Verification items for this drawing (mm, ordinates from the low corner). A direction names the side the tool comes from. Round coordinates to 2 decimals unless told otherwise and drop trailing zeros. Order: outer loops, then holes, each group sorted by start corner. A loop starts at its lowest first (then second) coordinate and runs counter-clockwise, first axis right, second up. Notation, with made-up numbers: (-25, -22.75) -> (16, -22.75) arc R13 cw to (16, -15.75) -> close; hole circle Ø1 at (-6, 81.5). An arc over 180 degrees is marked (long way). Answer in a Markdown table with one row per item. Add a question column.
1. Sectioned sample at C-C, the plane y = 10.5. Record the boundary of the cut face in (x, z), then the cut area to 3 significant figures.
2. Draft check along X on the marked faces 1, 2 and 3. Enter one of: +X half, -X half, draft (parallel to the pull), parting line (faces both ways), or undercut.
3. Depth check by flat-ended pin: P1, Ø7.5, axis at x = 53, y = 36, coming from the +Z side; P2, Ø1, axis at x = 38.5, z = 111.5, coming from the -Y side; P3, Ø6.5, axis at x = 69, y = 35, coming from the +Z side. Enter the tip coordinate at first touch or a pass-through.
4. Sectioned sample at B-B, the plane z = 98.5. Record the boundary of the cut face in (x, y), then the cut area to 3 significant figures.
5. Access from +Z, -Z, +X, -X, +Y, -Y to the whole of each face (thin tool, end or side, straight path). Record for the marked faces 4 and 5.
6. Material ranges on L1, parallel to X at y = 8.5, z = 69; L2, parallel to Z at x = 51, y = 37; L3, parallel to X at y = 24, z = 111.5, recorded low to high. Write a range as from..to.
7. Sectioned sample at A-A, the plane z = 118. Record the boundary of the cut face in (x, y), then the cut area to 3 significant figures.
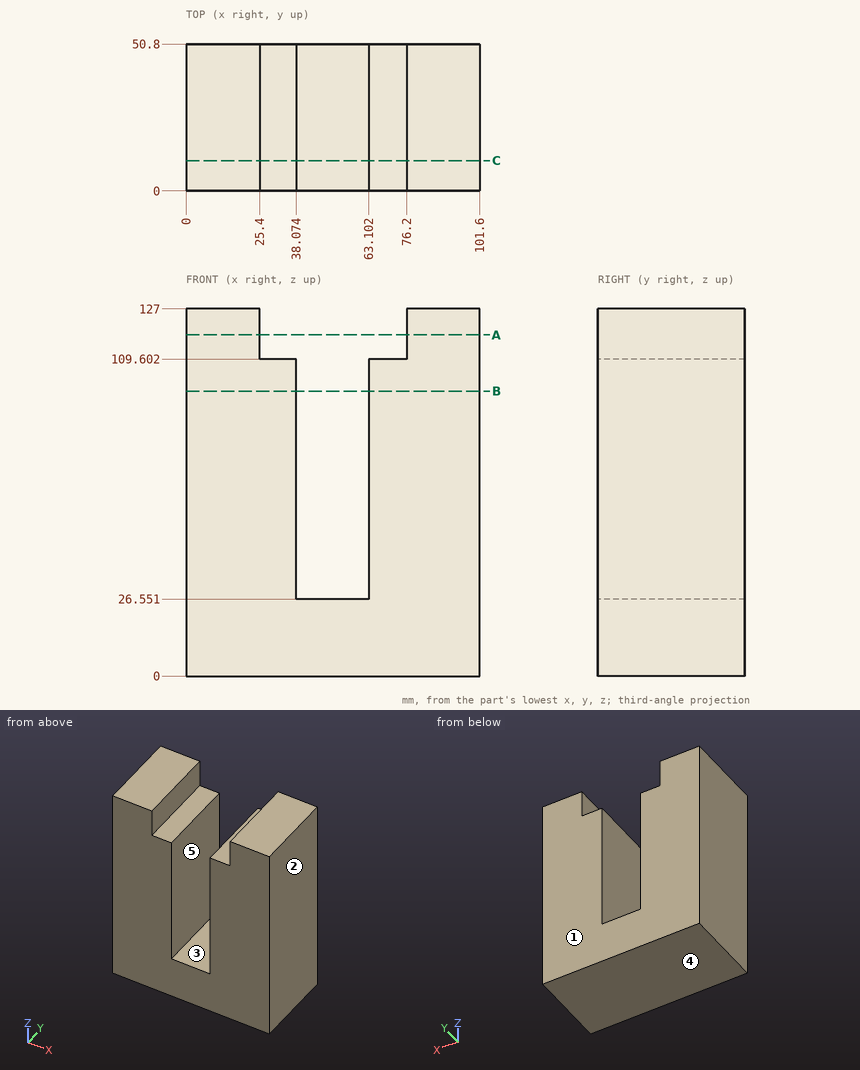
Answer key:
| question | item | result |
|---|---|---|
| 1 | outline | (0, 0) -> (101.6, 0) -> (101.6, 127) -> (76.2, 127) -> (76.2, 109.6) -> (63.1, 109.6) -> (63.1, 26.55) -> (38.07, 26.55) -> (38.07, 109.6) -> (25.4, 109.6) -> (25.4, 127) -> (0, 127) -> close |
| 1 | area | 9,940 mm² |
| 2 | face 1 | draft |
| 2 | face 2 | +X half |
| 2 | face 3 | undercut |
| 3 | P1 | stops at z = 26.55 |
| 3 | P2 | passes through |
| 3 | P3 | stops at z = 109.6 |
| 4 | outline | (0, 0) -> (38.07, 0) -> (38.07, 50.8) -> (0, 50.8) -> close; (63.1, 0) -> (101.6, 0) -> (101.6, 50.8) -> (63.1, 50.8) -> close |
| 4 | area | 3,890 mm² |
| 5 | face 4 | -Z, +X, -X, +Y, -Y |
| 5 | face 5 | +Z, +Y, -Y |
| 6 | L1 | x = 0..38.07, 63.1..101.6 |
| 6 | L2 | z = 0..26.55 |
| 6 | L3 | x = 0..25.4, 76.2..101.6 |
| 7 | outline | (0, 0) -> (25.4, 0) -> (25.4, 50.8) -> (0, 50.8) -> close; (76.2, 0) -> (101.6, 0) -> (101.6, 50.8) -> (76.2, 50.8) -> close |
| 7 | area | 2,580 mm² |
